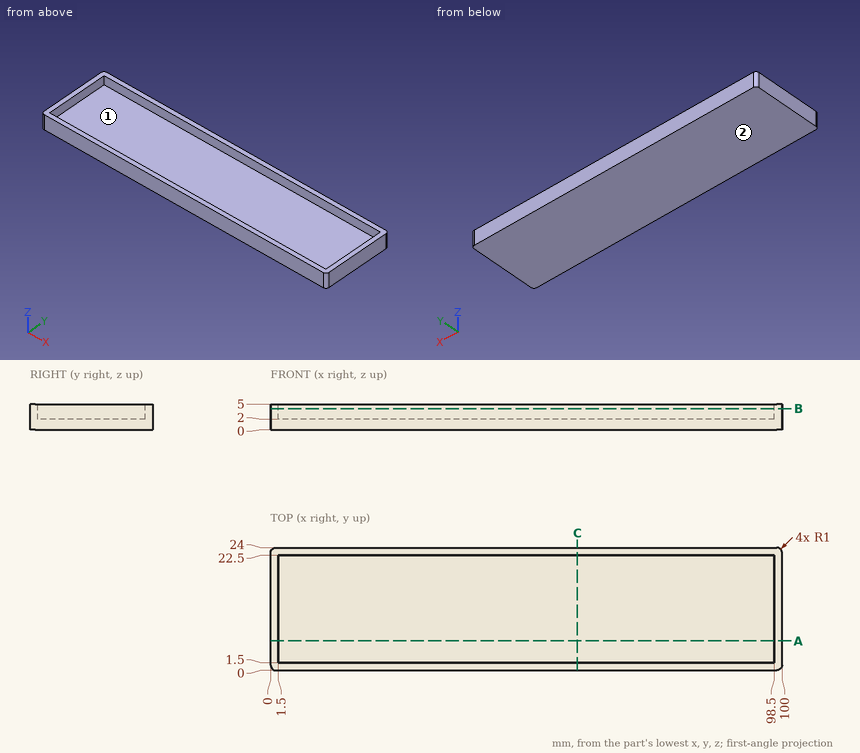
For this review, use the dimensioned drawing (mm, ordinates from the lowest corner) and the shaded views. Give positions to 0.01 mm unless a question says otherwise; leave off trailing zeros. Write each loop counter-clockwise with the first axis right and the second up, starting at its lowest first coordinate (ties: lowest second). Pieces come first, ordered by that corner, then holes. Notation, with made-up numbers: M -33.5,64.25 L 2.5,64.25 A19 cw 2.5,68.25 Z; hole C 22,44 d5. An arc over 180 degrees is marked long. Answer as a JSON object with one key per item and string values. Group by question number.
Item 1: Consider section B-B on z = 4.1. Write out the cut boundary in (x, y), plus the area to 3 significant figures.
Item 2: Consider section A-A on y = 5.75. Write out the cut boundary in (x, z).
Item 3: Draft analysis for pull direction Y (two halves, no side actions). For the marked faces 1 and 2, state which applies: +Y half, -Y half, draft (parallel to the pull), parting line (faces both ways), or undercut.
Item 4: For pin 1 Ø10.5 at (x, y) = (57.5, 15) entering from +Z, flat-tipped, find the tip position at first contact; note if it passes through.
Item 5: Consider section C-C on x = 60. Write out the cut boundary in (y, z), plus the area to 3 significant figures.
Item 6: For probe 1 along X at (y, z) = (18.5, 3.1); probe 2 along Y at (x, z) = (11, 2.7); probe 3 along Z at (x, y) = (63, 11.5), list the stretches that pass through material, from the lowest coordinate up. Write a range as [from, to].
Check result:
{
 "1": {"outline": "M 0,1 A1 ccw 1,0 L 99,0 A1 ccw 100,1 L 100,23 A1 ccw 99,24 L 1,24 A1 ccw 0,23 Z; hole M 1.5,1.5 L 98.5,1.5 L 98.5,22.5 L 1.5,22.5 Z", "area": "362 mm^2"},
 "2": {"outline": "M 0,0 L 100,0 L 100,5 L 98.5,5 L 98.5,2 L 1.5,2 L 1.5,5 L 0,5 Z"},
 "3": {"face 1": "undercut", "face 2": "draft"},
 "4": {"pin 1": "stops at z = 2"},
 "5": {"outline": "M 0,0 L 24,0 L 24,5 L 22.5,5 L 22.5,2 L 1.5,2 L 1.5,5 L 0,5 Z", "area": "57.0 mm^2"},
 "6": {"probe 1": "x = [0, 1.5], [98.5, 100]", "probe 2": "y = [0, 1.5], [22.5, 24]", "probe 3": "z = [0, 2]"}
}
